from build123d import *

# Parameters (mm, degrees)
F0_W     = 254
F0_H     = 4.7625
F3_DEPTH = 25.4
F4_R     = 2.54
F5_R     = 1.27


with BuildPart() as f1:
    # F0 (on Front) → F1 (revolve)
    with BuildSketch(Plane.XZ):
        with Locations((25.4, 2.38125)):
            Rectangle(F0_W, F0_H)
    revolve(axis=Axis((25.4, 0, 0), (1, 0, 0)))

    # F2 (on face) → F3 (cut)
    with BuildSketch(Plane.YZ.offset(152.4)):
        with BuildLine():
            ThreePointArc((3.781125, 2.8956), (0, 4.7625), (-3.781125, 2.8956))
            Line((-3.781125, 2.8956), (3.781125, 2.8956))
        make_face()
    extrude(amount=-F3_DEPTH, mode=Mode.SUBTRACT)

    # F4
    f4_edges = [f1.edges().sort_by_distance(p)[0] for p in [
        (-101.6, 0, -4.7625),
    ]]
    fillet(f4_edges, radius=F4_R)

    # F5
    f5_edges = [f1.edges().sort_by_distance(p)[0] for p in [
        (152.4, 0, -4.7625),
    ]]
    fillet(f5_edges, radius=F5_R)


solid = f1.part
Geometry: final body of the model. Coordinates: model frame, mm. A direction names the side the tool comes from. Coordinates: 2 decimals unless noted, no trailing zeros. Order: outer loops, then holes, each group sorted by start corner. A loop starts at its lowest first (then second) coordinate and runs counter-clockwise, first axis right, second up. Notation, with made-up numbers: (39, 82) - (73, 82) arc R27 ccw to (73, 116) - close; hole circle Ø10 at (-21, 18). An arc over 180 degrees is marked (long way). Use one line per item in the form item = value.
1) Ray query, L1, parallel to X at y = 2.5, z = 1; L2, parallel to X at y = -3.5, z = -2.5; L3, parallel to Y at x = -8.5, z = -1. Return the intervals inside material, ascending.
Solutions:
L1 = -101.56 to 152.4
L2 = -100.52 to 152.11
L3 = -4.66 to 4.66
2) Section A-A (x = -21). Return loops of the section in (y, z) (1 decimal), then the cut area to 3 significant figures.
Solutions:
outline = circle Ø9.5 at (0, 0)
area = 71.3 mm^2
3) Pin query (flat end, axial travel): pin 1 (2 mm diameter, centred on y = 0.5, z = 4, fed in from +X); pin 2 (1.5 mm diameter, centred on x = 6.5, y = 1, fed in from -Z); pin 3 (2 mm diameter, centred on x = 104, z = -3.5, fed in from -Y). Return the tip coordinate at first contact, or that it passes through.
Solutions:
pin_1 = 127
pin_2 = -4.76
pin_3 = -4.05
4) Set-up query: faces 1 (the face through (140, 0, 2.896)), 2 (the face through (-101.6, 0, 0)). Return all of +Z, -Z, +X, -X, +Y, -Y with unobstructed straight access to the full face (end or side cutting, diameter ignored); none if empty.
Solutions:
face_1 = +Z, +X, +Y, -Y
face_2 = +Z, -Z, -X, +Y, -Y
